Part model, mm, in its own coordinate system. Coordinates: 2 decimals unless noted, no trailing zeros. Write each loop counter-clockwise with the first axis right and the second up, starting at its lowest first coordinate (ties: lowest second). Pieces come first, ordered by that corner, then holes. Notation, with made-up numbers: (83.25, 7.5) -> (90.25, 7.5) arc R19 ccw to (90.25, 18.5) -> close; hole circle Ø4 at (26, 84). An arc over 180 degrees is marked (long way). Write item = value, one per line. Start each with the question number.
Q1. Probe line 1 (Y direction, x = -120, z = 1.85); line 2 (Y direction, x = -113.5, z = 2.3); line 3 (Y direction, x = -83.5, z = 1.7). List the from-to ranges inside material, lowest first.
Q2. Band-saw the part on A-A, the plane x = 172. List the corners of the cut face in (y, z).
Q3. Pull direction Y, two halves, no side cores. Call faces 1 (the cylindrical face through (-4.23, 22.94, 1.52)), 2 (the cylindrical face through (204.78, 0.63, 1.48)), 3 (the flat face through (-56, 22, 3)): released by +Y, released by -Y, zero draft, split by the parting line, or undercut.
Q4. Band-saw the part on C-C, the plane x = 98. List the corners of the cut face in (y, z), plus the area to 3 significant figures.
Q5. Band-saw the part on B-B, the plane x = -76.5. List the corners of the cut face in (y, z).
Q6. Band-saw the part on D-D, the plane z = 0.6. Give the number of separate pieces and of enclosed holes in the cut face, plus the area to 3 significant figures.
from build123d import *

# Parameters (mm, degrees)
SKETCH1_R               = 11.1125
SKETCH1_R_2             = 1.6
BOSS_EXTRUDE1_DEPTH     = 3
M3_CLEARANCE_HOLE1_D    = 3.4
CUT_EXTRUDE1_DEPTH      = 10
SKETCH10_R              = 1.6
BOSS_EXTRUDE3_DEPTH     = 3
CUT_EXTRUDE2_DEPTH      = 231.98836087
CUT_EXTRUDE2_DEPTH_BACK = 231.98836087


with BuildPart() as part:
    # Sketch1 → Boss-Extrude1 (new body)
    with BuildSketch(Plane.XY):
        with BuildLine():
            Line((-172.112162162, 49.916534261), (176.720292805, 29.735414369))
            ThreePointArc((176.720292805, 29.735414369), (204.785135135, 0), (176.720292805, -29.735414369))
            Line((176.720292805, -29.735414369), (-172.112162162, -49.916534261))
            ThreePointArc((-172.112162162, -49.916534261), (-225, 0), (-172.112162162, 49.916534261))
        make_face()
        with Locations((175, 0)):
            Circle(SKETCH1_R, mode=Mode.SUBTRACT)
        with Locations((-175, 0)):
            Circle(SKETCH1_R, mode=Mode.SUBTRACT)
        with Locations((-120, 41.392475449)):
            Circle(SKETCH1_R_2, mode=Mode.SUBTRACT)
        with Locations((-55.108505461, 37.63828626)):
            Circle(SKETCH1_R_2, mode=Mode.SUBTRACT)
        with Locations((9.782989078, 33.884097071)):
            Circle(SKETCH1_R_2, mode=Mode.SUBTRACT)
        with Locations((74.674483618, 30.129907882)):
            Circle(SKETCH1_R_2, mode=Mode.SUBTRACT)
        with Locations((139.565978157, 26.375718693)):
            Circle(SKETCH1_R_2, mode=Mode.SUBTRACT)
        with Locations(Location((139.565978157, -26.375718693, 0), (0, 0, 180))):
            Circle(SKETCH1_R_2, mode=Mode.SUBTRACT)
        with Locations(Location((74.674483618, -30.129907882, 0), (0, 0, 180))):
            Circle(SKETCH1_R_2, mode=Mode.SUBTRACT)
        with Locations(Location((9.782989078, -33.884097071, 0), (0, 0, 180))):
            Circle(SKETCH1_R_2, mode=Mode.SUBTRACT)
        with Locations(Location((-55.108505461, -37.63828626, 0), (0, 0, 180))):
            Circle(SKETCH1_R_2, mode=Mode.SUBTRACT)
        with Locations(Location((-120, -41.392475449, 0), (0, 0, 180))):
            Circle(SKETCH1_R_2, mode=Mode.SUBTRACT)
        with Locations((-87.55425273, 39.515380855)):
            Circle(SKETCH1_R_2, mode=Mode.SUBTRACT)
        with Locations((-165.112162162, -44.002364352)):
            Circle(SKETCH1_R_2, mode=Mode.SUBTRACT)
        with Locations(Location((-165.112162162, 44.002364352, 0), (0, 0, 180))):
            Circle(SKETCH1_R_2, mode=Mode.SUBTRACT)
        with Locations((132.57766336, -26.78001599)):
            Circle(SKETCH1_R_2, mode=Mode.SUBTRACT)
    extrude(amount=BOSS_EXTRUDE1_DEPTH)

    # M3 Clearance Hole1 (through all)
    with Locations(Plane.XY.offset(3)):
        with Locations((-197.5, 0), (-175, 22.5), (-152.5, 0), (-175, -22.5)):
            Hole(M3_CLEARANCE_HOLE1_D / 2)

    # Sketch7 → Cut-Extrude1 (cut)
    with BuildSketch(Plane.XY.offset(3)):
        with BuildLine():
            Line((88.975526403, 22.70262828), (139.057512253, 7.661932008))
            ThreePointArc((139.057512253, 7.661932008), (144.756469468, 0), (139.057512253, -7.661932008))
            Line((139.057512253, -7.661932008), (88.975526403, -22.70262828))
            ThreePointArc((88.975526403, -22.70262828), (81.899985858, -21.459743798), (78.674483618, -15.040696272))
            Line((78.674483618, -15.040696272), (78.674483618, 15.040696272))
            ThreePointArc((78.674483618, 15.040696272), (81.899985858, 21.459743798), (88.975526403, 22.70262828))
        make_face()
        with BuildLine():
            Line((70.674483618, -1.435965036), (70.674483618, 18.804082595))
            ThreePointArc((70.674483618, 18.804082595), (68.492405602, 24.295146589), (63.136537672, 26.790728077))
            Line((63.136537672, 26.790728077), (41.340803255, 28.05168394))
            ThreePointArc((41.340803255, 28.05168394), (33.5681452, 23.313895048), (35.260532637, 14.369808645))
            Line((35.260532637, 14.369808645), (57.056267053, -7.13119485))
            ThreePointArc((57.056267053, -7.13119485), (65.761089155, -8.816538609), (70.674483618, -1.435965036))
        make_face()
        with BuildLine():
            Line((29.274282074, 9.037636121), (52.642195402, -14.014286633))
            ThreePointArc((52.642195402, -14.014286633), (54.510022559, -22.530712895), (47.486032892, -27.696161929))
            Line((47.486032892, -27.696161929), (25.525253015, -28.966666222))
            ThreePointArc((25.525253015, -28.966666222), (19.742509337, -26.954153474), (17.076553479, -21.442074794))
            Line((17.076553479, -21.442074794), (15.669420028, 2.880352253))
            ThreePointArc((15.669420028, 2.880352253), (20.357520369, 10.630725727), (29.274282074, 9.037636121))
        make_face()
        with BuildLine():
            Line((0.769210605, -16.592065878), (-1.180512913, 17.109078816))
            ThreePointArc((-1.180512913, 17.109078816), (-4.302872031, 22.998301654), (-10.802267436, 24.478143355))
            Line((-10.802267436, 24.478143355), (-90.530788222, 7.831118593))
            ThreePointArc((-90.530788222, 7.831118593), (-96.895679181, 0), (-90.530788222, -7.831118593))
            Line((-90.530788222, -7.831118593), (-8.852543917, -24.885238525))
            ThreePointArc((-8.852543917, -24.885238525), (-1.994439382, -23.113849139), (0.769210605, -16.592065878))
        make_face()
        with BuildLine():
            Line((5.567875781, -14.698862148), (4.412740646, 5.267751556))
            ThreePointArc((4.412740646, 5.267751556), (7.328519824, 8.541622626), (10.602390894, 5.625843448))
            Line((10.602390894, 5.625843448), (11.757526029, -14.340770256))
            ThreePointArc((11.757526029, -14.340770256), (8.841746851, -17.614641327), (5.567875781, -14.698862148))
        make_face()
        with BuildLine():
            Line((-126.896651592, 21.273781799), (-116.432051872, 34.601649091))
            ThreePointArc((-116.432051872, 34.601649091), (-114.179639962, 36.365789869), (-111.366346547, 36.886301404))
            Line((-111.366346547, 36.886301404), (-69.577822511, 34.468696042))
            ThreePointArc((-69.577822511, 34.468696042), (-63.940794692, 28.922456993), (-68.698031271, 22.605372985))
            Line((-68.698031271, 22.605372985), (-120.951155027, 11.695111055))
            ThreePointArc((-120.951155027, 11.695111055), (-127.275300447, 14.404228754), (-126.896651592, 21.273781799))
        make_face()
        with BuildLine():
            Line((-111.366346547, -36.886301404), (-69.577822511, -34.468696042))
            ThreePointArc((-69.577822511, -34.468696042), (-63.940794692, -28.922456993), (-68.698031271, -22.605372985))
            Line((-68.698031271, -22.605372985), (-120.951155027, -11.695111055))
            ThreePointArc((-120.951155027, -11.695111055), (-127.275300447, -14.404228754), (-126.896651592, -21.273781799))
            Line((-126.896651592, -21.273781799), (-116.432051872, -34.601649091))
            ThreePointArc((-116.432051872, -34.601649091), (-114.179639962, -36.365789869), (-111.366346547, -36.886301404))
        make_face()
    extrude(amount=-CUT_EXTRUDE1_DEPTH, mode=Mode.SUBTRACT)

    # Sketch10 → Boss-Extrude3 (add)
    with BuildSketch(Plane.XY.offset(3)):
        with BuildLine():
            Line((-172.112162162, 49.916534261), (-210.904992847, 52.160828781))
            ThreePointArc((-210.904992847, 52.160828781), (-214.519207646, 50.903008313), (-216.185430057, 47.457959138))
            Line((-216.185430057, 47.457959138), (-217.397717482, 26.503463026))
            Line((-217.397717482, 26.503463026), (-172.112162162, 49.916534261))
        make_face()
        with Locations((-210.224324324, 46.612253255)):
            Circle(SKETCH10_R, mode=Mode.SUBTRACT)
    boss_extrude3 = extrude(amount=-BOSS_EXTRUDE3_DEPTH)

    # Mirror1: Boss-Extrude3 across plane
    add(boss_extrude3.mirror(Plane.ZX))

    # Sketch11 → Cut-Extrude2 (cut, two sides: drawn at the far end of the back side and taken through both)
    with BuildSketch(Plane(origin=(0, 0, 0), x_dir=(-1, 0, 0), z_dir=(0, 0, -1)).offset(-CUT_EXTRUDE2_DEPTH_BACK)):
        with BuildLine():
            Line((217.397717482, -26.503463026), (217.397717482, 26.503463026))
            ThreePointArc((217.397717482, 26.503463026), (225, 0), (217.397717482, -26.503463026))
        make_face()
    extrude(amount=CUT_EXTRUDE2_DEPTH + CUT_EXTRUDE2_DEPTH_BACK, mode=Mode.SUBTRACT)


solid = part.part
Ans:
q1.line_1 = -46.9 to -42.99, -39.79 to -30.06, -11.89 to 11.89, 30.06 to 39.79, 42.99 to 46.9
q1.line_2 = -46.53 to -36.62, -13.25 to 13.25, 36.62 to 46.53
q1.line_3 = -44.79 to -35.27, -19.51 to -9.3, 9.3 to 19.51, 35.27 to 44.79
q2.outline = (-30.01, 0) -> (-10.7, 0) -> (-10.7, 3) -> (-30.01, 3) -> close; (10.7, 0) -> (30.01, 0) -> (30.01, 3) -> (10.7, 3) -> close
q3.face_1 = undercut
q3.face_2 = split by the parting line
q3.face_3 = zero draft
q4.outline = (-34.29, 0) -> (-19.99, 0) -> (-19.99, 3) -> (-34.29, 3) -> close; (19.99, 0) -> (34.29, 0) -> (34.29, 3) -> (19.99, 3) -> close
q4.area = 85.8 mm2
q5.outline = (-44.39, 0) -> (-34.87, 0) -> (-34.87, 3) -> (-44.39, 3) -> close; (-20.98, 0) -> (-10.76, 0) -> (-10.76, 3) -> (-20.98, 3) -> close; (10.76, 0) -> (20.98, 0) -> (20.98, 3) -> (10.76, 3) -> close; (34.87, 0) -> (44.39, 0) -> (44.39, 3) -> (34.87, 3) -> close
q6.separate_pieces = 1
q6.enclosed_holes = 29
q6.area = 23,100 mm2
